Read the model definition and answer for the solid it produces. Units are mm, in the model's axes. Face numbers are marked on the shaded views. A direction names the side the tool comes from. Coordinates: 2 decimals unless noted, no trailing zeros. Loops run counter-clockwise (first coordinate to the right, second up) from the corner with the lowest first, then second, coordinate; pieces in that order, holes last. Notation, with made-up numbers: M 42,51.25 L 82,51.25 A22 cw 82,58.25 Z; hole C -30,49.5 d6. An arc over 180 degrees is marked long. One line per item, written item: value. Start each with the question number.
1. The part is cut by section B-B (x = 24). Write down the section's boundary in (y, z) (3 decimals).
2. Consider probe 1 along Y at (x, z) = (25, -15) (3 decimals); probe 2 along Y at (x, z) = (27, -15) (3 decimals); probe 3 along Z at (x, y) = (26, 23.56). Determine where each line is inside the solid, lowest interval first.
3. Flat-ended cylindrical pins translate along their axes: pin 1 (1.5 mm diameter, centred on x = 22, z = -23, fed in from +Y); pin 2 (4.5 mm diameter, centred on x = 7.5, z = -34.5, fed in from -Y); pin 3 (8 mm diameter, centred on x = 24.5, y = -7.5, fed in from +Z) (3 decimals). Find the tip coordinate at first contact, or state that the pin passes through.
4. The part is cut by section C-C (z = -15). State how many separate pieces and enclosed holes the cut face has, then the cut area to 3 significant figures.
5. The part is cut by section A-A (y = 23.56). Write down the section's boundary in (x, z), then the cut area to 3 significant figures.
6. For the marked faces 1, 2, 3, 4 and 5, determine the directions among +Z, -Z, +X, -X, +Y, -Y from which every point of the face is accessible in a straight line to the end or side of a thin tool.
7. The part is cut by section D-D (z = 2). Write down the section's boundary in (x, y), then the cut area to 3 significant figures.
8. Determine the mould class of the marked faces 6, 7 and 8 for opening direction Z: +Z half, -Z half, draft (parallel to the pull), parting line (faces both ways), or undercut.
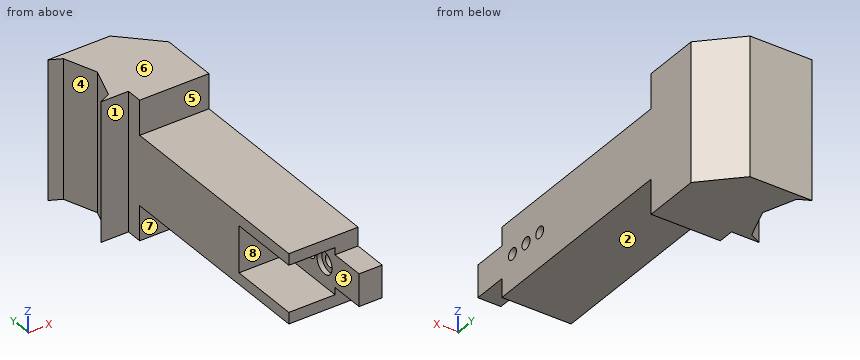
Autodesk Inventor part; units mm, degrees
ref_plane "Work Plane1" through (0, 0, -15) normal (0, 0, 1) x (1, 0, 0)
ref_plane "YZ Plane" through (0, 0, 0) normal (1, 0, 0) x (0, 1, 0)
ref_plane "XZ Plane" through (0, 0, 0) normal (0, 1, 0) x (-1, 0, 0)
sketch "Sketch1" plane through (0, 0, 0) normal (0, 0, 1) x (1, 0, 0)
  line L0 (0, 0) -> (25, 0)
  line L1 (25, 0) -> (25, 40)
  line L2 (25, 40) -> (0, 40)
  line L3 (0, 40) -> (0, 0)
  dimension "d1" = 25
  dimension "d2" = 40
  dimension "d3" = 25
extrude "Extrusion1" add sketch "Sketch1" against normal blind 30
sketch "Sketch2" plane through (25, 0, 0) normal (1, 0, 0) x (0, 0, -1)
  line L0 (0, 0) -> (30, 0)
  circle A0 centre (15, 6.56) radius 2.46
extrude "Extrusion2" cut sketch "Sketch2" against normal blind 30
sketch "Sketch3" plane through (0, 0, 0) normal (-1, 0, 0) x (0, 0, 1)
  line L0 (0, 0) -> (-30, 0)
  line L1 (-25.05, 0) -> (-4.95, 0)
  line L2 (-4.95, 0) -> (-4.95, 33.12)
  line L3 (-4.95, 33.12) -> (-25.05, 33.12)
  line L4 (-25.05, 33.12) -> (-25.05, 0)
  dimension "d11" = 20.1
extrude "Extrusion3" cut sketch "Sketch3" against normal blind 20
sketch "Sketch4" plane through (0, 0, 0) normal (0, -1, 0) x (1, 0, 0)
  line L0 (20, -4.95) -> (20, -25.05)
  line L1 (20, -15) -> (25, -15)
  line L2 (25, 0) -> (25, -30)
  line L3 (20, -8.025) -> (25, -8.025)
  line L4 (25, -8.025) -> (25, -21.975)
  line L5 (25, -21.975) -> (20, -21.975)
  line L6 (20, -21.975) -> (20, -8.025)
  line L7 (20, -8.025) -> (25, -21.975) construction
  line L8 (25, -8.025) -> (20, -21.975) construction
  line L9 (25, -12.54) -> (25, -17.46)
  point P0 (0, 0)
  point P1 (22.5, -15)
  dimension "d14" = 13.95
extrude "Extrusion4" add sketch "Sketch4" along normal blind 15
sketch "Sketch5" plane through (20, 0, 0) normal (-1, 0, 0) x (0, 0, 1)
  circle A0 centre (-15, 6.56) radius 2.46
  circle A1 centre (-15, 6.56) radius 4.7025
  circle A2 centre (-15, 6.56) radius 2.46
  circle A3 centre (-15, 6.56) radius 2.46
  point P0 (0, 0)
  dimension "d17" = 9.405
extrude "Extrusion5" cut sketch "Sketch5" against normal blind 2.1
sketch "Sketch6" plane through (25, 0, 0) normal (1, 0, 0) x (0, 0, -1)
  circle A0 centre (15, 6.56) radius 4.7025
  line L0 (15, 6.56) -> (15, 23.56)
  circle A1 centre (15, 23.56) radius 2.46
  point P0 (0, 0)
  dimension "d20" = 17
  dimension "d21" = 4.92
extrude "Extrusion6" cut sketch "Sketch6" against normal blind 10 contours A1
sketch "Sketch7" plane through (20, 0, 0) normal (-1, 0, 0) x (0, 0, 1)
  circle A0 centre (-15, 23.56) radius 2.46
  circle A1 centre (-15, 23.56) radius 4.7025
  point P0 (0, 0)
  dimension "d24" = 9.405
extrude "Extrusion7" cut sketch "Sketch7" against normal blind 2.1
sketch "Sketch9" plane through (25, 0, 0) normal (1, 0, 0) x (0, 0, -1)
  circle A0 centre (15, 6.56) radius 2.46
  circle A1 centre (15, 6.56) radius 2.46
  circle A2 centre (15, 23.56) radius 2.46
  circle A3 centre (15, 23.56) radius 2.46
  line L0 (30, 40) -> (30, 0)
  line L1 (30, 0) -> (30, 40)
  line L2 (30, 40) -> (0, 40)
  line L3 (0, 40) -> (0, 0)
  line L4 (0, 0) -> (8.025, 0)
  line L5 (21.975, 0) -> (21.975, -15)
  line L6 (21.975, -15) -> (8.025, -15)
  line L7 (8.025, -15) -> (8.025, 0)
  line L8 (0, 0) -> (8.025, 0)
  line L9 (21.975, 0) -> (30, 0)
extrude "Extrusion8" add sketch "Sketch9" along normal blind 5
sketch "Sketch10" plane through (0, 40, 0) normal (0, 1, 0) x (1, 0, 0)
  line L0 (0, 30) -> (30, 30)
  line L1 (30, 0) -> (0, 0)
  line L2 (0, 30) -> (30, 30)
  line L3 (30, 30) -> (30, 0)
  line L4 (30, 0) -> (0, 0)
  line L5 (0, 0) -> (0, 30)
extrude "Extrusion9" add sketch "Sketch10" along normal blind 30
sketch "Sketch12" plane through (30, 0, 0) normal (1, 0, 0) x (0, 0, -1)
  circle A0 centre (15, 6.56) radius 2.46
  line L0 (15, 6.56) -> (15, 15.06)
  circle A1 centre (15, 15.06) radius 2.525
  point P0 (0, 0)
  dimension "d31" = 8.5
  dimension "d33" = 5.05
extrude "Extrusion10" cut sketch "Sketch12" against normal blind 30 contours A1
sketch "Sketch14" plane through (0, 0, 0) normal (0, 0, 1) x (1, 0, 0)
  line L0 (30, 70) -> (0, 70)
  line L1 (0, 70) -> (0, 85)
  line L2 (30, 0) -> (30, 70)
  line L3 (30, 118) -> (30, 70)
  line L4 (30, 105) -> (30, 100)
  line L5 (-12, 133) -> (15, 133)
  line L6 (-7, 130.5) -> (-12, 133)
  line L7 (-7, 130.5) -> (-2, 116.5)
  line L8 (-7, 102.5) -> (-12, 100)
  line L9 (-7, 102.5) -> (-2, 116.5)
  line L10 (30, 118) -> (15, 133)
  line L11 (0, 100) -> (-12, 100)
  line L12 (0, 100) -> (0, 85)
  point P0 (0, 0)
  dimension "d79" = 12
extrude "Extrusion12" add sketch "Sketch14" against normal blind 30
sketch "Sketch15" plane through (0, 0, -25.05) normal (-1, 0, 0) x (0, 0, 1)
  line L0 (0, 33.12) -> (20.1, 33.12)
  line L1 (20.1, 33.12) -> (20.1, 0)
  line L2 (0, 33.12) -> (20.1, 33.12)
  line L3 (20.1, 33.12) -> (20.1, 31.1)
  line L4 (20.1, 31.1) -> (0, 31.1)
  line L5 (0, 31.1) -> (0, 33.12)
  point P0 (25.05, 0)
  dimension "d57" = 2.02
extrude "Extrusion13" add sketch "Sketch15" against normal blind 20
sketch "Sketch22" plane through (0, 0, 0) normal (0, 0, 1) x (1, 0, 0)
  line L0 (0, 100) -> (-12, 100)
  line L1 (0, 100) -> (-12, 100)
  line L2 (-12, 100) -> (-7, 102.5)
  line L3 (-12, 100) -> (-7, 102.5)
  line L4 (-7, 102.5) -> (-2, 116.5)
  line L5 (-7, 102.5) -> (-2, 116.5)
  line L6 (-2, 116.5) -> (-7, 130.5)
  line L7 (-2, 116.5) -> (-7, 130.5)
  line L8 (-7, 130.5) -> (-12, 133)
  line L9 (-7, 130.5) -> (-12, 133)
  line L10 (-12, 133) -> (15, 133)
  line L11 (-12, 133) -> (15, 133)
  line L12 (15, 133) -> (30, 118)
  line L13 (15, 133) -> (30, 118)
  line L14 (30, 118) -> (30, 93)
  line L15 (30, 0) -> (30, 118)
  line L16 (30, 93) -> (0, 93)
  line L17 (0, 100) -> (0, 0)
  line L18 (0, 93) -> (0, 100)
  dimension "d80" = 25
extrude "Extrusion14" add sketch "Sketch22" along normal blind 15
ref_plane "Work Plane1" through (0, 0, -15) normal (0, 0, 1) x (1, 0, 0)
mirror "Mirror1" about plane through (0, 0, -15) normal (0, 0, 1) of "Extrusion14"
properties part number "rec_b_28mm_x_60mm"
Answer block:
1. outline: M -15,-21.975 L 0,-21.975 L 0,-30 L 93,-30 L 93,-45 L 124,-45 L 124,15 L 93,15 L 93,0 L 0,0 L 0,-8.025 L -15,-8.025 Z; hole C 6.56,-15 d4.92; hole C 15.06,-15 d5.05; hole C 23.56,-15 d4.92
2. probe 1: y = -15 to 4.1, 9.02 to 12.535, 17.585 to 21.1, 26.02 to 123
2. probe 2: y = -15 to 4.1, 9.02 to 12.535, 17.585 to 21.1, 26.02 to 121
2. probe 3: z = -30 to -17.46, -12.54 to 0
3. pin 1: stops at y = 126.75
3. pin 2: stops at y = 93
3. pin 3: stops at z = -8.025
4. separate pieces: 4
4. enclosed holes: 0
4. area: 3,410 mm2
5. outline: M 0,-30 L 30,-30 L 30,-17.46 L 22.1,-17.46 L 22.1,-19.7 L 20,-19.7 L 20,-25.05 L 0,-25.05 Z; M 0,-4.95 L 20,-4.95 L 20,-10.3 L 22.1,-10.3 L 22.1,-12.54 L 30,-12.54 L 30,0 L 0,0 Z
5. area: 439 mm2
6. face 1: +Z, -Z, -X, -Y
6. face 2: -Z, +X, -X, -Y
6. face 3: -X, -Y
6. face 4: +Z, -Z, -X
6. face 5: +Z, +X, -X, -Y
7. outline: M -12,100 L 0,100 L 0,93 L 30,93 L 30,118 L 15,133 L -12,133 L -7,130.5 L -2,116.5 L -7,102.5 Z
7. area: 1,260 mm2
8. face 6: +Z half
8. face 7: draft
8. face 8: undercut
